Autodesk Inventor part; units mm, degrees
ref_plane "YZ Plane" through (0, 0, 0) normal (1, 0, 0) x (0, 1, 0)
ref_plane "XZ Plane" through (0, 0, 0) normal (0, 1, 0) x (-1, 0, 0)
ref_plane "XY Plane" through (0, 0, 0) normal (0, 0, 1) x (1, 0, 0)
sketch "Sketch1" plane through (0, 0, 0) normal (0, 1, 0) x (-1, 0, 0)
  line L0 (3.5, 2.0207) -> (0, 4.0415)
  line L1 (0, 4.0415) -> (-3.5, 2.0207)
  line L2 (-3.5, 2.0207) -> (-3.5, -2.0207)
  line L3 (-3.5, -2.0207) -> (0, -4.0415)
  line L4 (-4.4202, 8.8438) -> (-5.8936, 1.125)
  arc A0 (4.4202, 8.8438) -> (-4.4202, 8.8438) centre (0, 8) ccw
  line L5 (5.8936, 1.125) -> (4.4202, 8.8438)
  line L6 (0, -4.0415) -> (3.5, -2.0207)
  arc A1 (-5.8936, 1.125) -> (5.8936, 1.125) centre (0, 0) ccw
  line L7 (3.5, -2.0207) -> (3.5, 2.0207)
extrude "Extrusion1" add sketch "Sketch1" along normal blind 5
sketch "Sketch2" plane through (0, 5, 0) normal (0, 1, 0) x (1, 0, 0)
  point P0 (0, -8)
hole "Hole1" at (0, 5, 8) direction (0, -1, 0) diameter 4.5 depth 5
properties part number "Piston Nut trap" material "ASA Plastic"
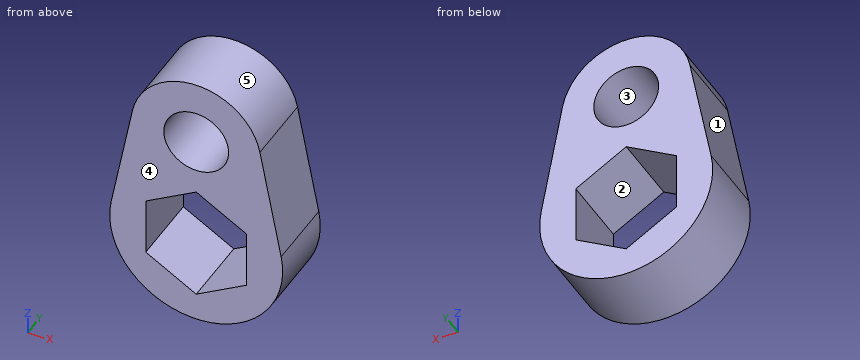
Can you work these out from the model? Positions are in its coordinate system, mm. Face numbers are marked on the shaded views. A direction names the side the tool comes from. Coordinates: 2 decimals unless noted, no trailing zeros. Loops run counter-clockwise (first coordinate to the right, second up) from the corner with the lowest first, then second, coordinate; pieces in that order, holes last. Notation, with made-up numbers: M 2.25,64.25 L 18.25,64.25 A34 cw 18.25,95.25 Z; hole C 30.5,-7.5 d11. An arc over 180 degrees is marked long. Put each result on its own line as item: value. Start each with the question number.
(1) Imagine slicing it at A-A on y = 4.6. Give the number of separate pieces and of enclosed holes in the cut face, and give its area (3 significant figures).
(2) Will these pins go through, and if not, where does the flat tip stop? pin 1 Ø3 at (y, z) = (2.5, -0.5) entering from -X; pin 2 Ø1.5 at (y, z) = (0.5, -3.5) entering from +X; pin 3 Ø2.5 at (x, z) = (0, 8) entering from -Y; pin 4 Ø1 at (x, y) = (4.5, 4) entering from -Z.
(3) Imagine slicing it at C-C on x = -3. List the corners of the cut face in (y, z) for me, and give its area (3 significant figures).
(4) I need wall thicknesses on probe 1 along Z at (x, y) = (-2, 0.45); probe 2 along Z at (x, y) = (-0.5, 4.65); probe 3 along X at (y, z) = (3.3, 8). Which ranges of each line are inside material? Lowest first, please.
(5) Imagine slicing it at D-D on x = -1. List the corners of the cut face in (y, z) for me, and give its area (3 significant figures).
(6) Which directions (+Z, -Z, +X, -X, +Y, -Y) give clear straight access to the entire face, cutting with the end or side of a thin tool? Please do the marked faces 1 and 2.
(7) We'd pull the mould along Z, two halves only. Please class the marked faces 3, 4 and 5: +Z half, -Z half, draft (parallel to the pull), parting line (faces both ways), or undercut.
(8) Imagine slicing it at B-B on z = 0. List the corners of the cut face in (x, y) for me.
Worked answers:
1. separate pieces: 1
1. enclosed holes: 2
1. area: 115 mm2
2. pin 1: stops at x = -6
2. pin 2: stops at x = 5.33
2. pin 3: passes through
2. pin 4: stops at z = -4.47
3. outline: M 0,-5.2 L 5,-5.2 L 5,-2.31 L 0,-2.31 Z; M 0,2.31 L 5,2.31 L 5,11.35 L 0,11.35 Z
3. area: 59.7 mm2
4. probe 1: z = -5.66 to -2.89, 2.89 to 6.97, 9.03 to 12.03
4. probe 2: z = -5.98 to -3.75, 3.75 to 5.81, 10.19 to 12.47
4. probe 3: x = -4.58 to -2.25, 2.25 to 4.58
5. outline: M 0,-5.92 L 5,-5.92 L 5,-3.46 L 0,-3.46 Z; M 0,3.46 L 5,3.46 L 5,5.98 L 0,5.98 Z; M 0,10.02 L 5,10.02 L 5,12.39 L 0,12.39 Z
5. area: 36.7 mm2
6. face 1: +Z, -X, +Y, -Y
6. face 2: +Y, -Y
7. face 3: undercut
7. face 4: draft
7. face 5: +Z half
8. outline: M -6,0 L -3.5,0 L -3.5,5 L -6,5 Z; M 3.5,0 L 6,0 L 6,5 L 3.5,5 Z
